```python
from build123d import *

# Parameters (mm, degrees)
F0_R     = 10
F2_DEPTH = 10
F1_R     = 6.465
F3_DEPTH = 12
F4_R     = 6.465
F6_DEPTH = 2
F7_D     = 10
F8_SIZE2 = 2
F8_SIZE  = 2
F9_SIZE2 = 0.5
F9_SIZE  = 0.5


with BuildPart() as f2:
    # F0 (on Top) → F2 (new body)
    with BuildSketch(Plane.XY):
        Circle(F0_R)
    extrude(amount=F2_DEPTH)

    # F1 (on Top) → F3 (cut)
    with BuildSketch(Plane.XY):
        Circle(F1_R)
    extrude(amount=F3_DEPTH, mode=Mode.SUBTRACT)

    # F4 (on face) → F6 (join)
    with BuildSketch(Plane.XY):
        Circle(F4_R)
    extrude(amount=F6_DEPTH)

    # F7 (through all)
    with Locations(Plane(origin=(0, 0, 0), x_dir=(1, 0, 0), z_dir=(0, 0, -1))):
        with Locations((0, 0)):
            Hole(F7_D / 2)

    # F8
    f8_edges = [f2.edges().sort_by_distance(p)[0] for p in [
        (-10, 0, 10),
        (-10, 0, 0),
    ]]
    chamfer(f8_edges, length=F8_SIZE, length2=F8_SIZE2)

    # F9
    f9_edges = [f2.edges().sort_by_distance(p)[0] for p in [
        (-6.465, 0, 10),
    ]]
    chamfer(f9_edges, length=F9_SIZE, length2=F9_SIZE2)


solid = f2.part
```
Here's how the part is built. I have some questions about the finished solid (model axes, mm). A direction names the side the tool comes from. Coordinates: 2 decimals unless noted, no trailing zeros. Order: outer loops, then holes, each group sorted by start corner. A loop starts at its lowest first (then second) coordinate and runs counter-clockwise, first axis right, second up. Notation, with made-up numbers: (-33.75, 18) - (1.25, 18) arc R29 ccw to (1.25, 42) - close; hole circle Ø6 at (41, -2.5). An arc over 180 degrees is marked (long way). One line per question, with ' | ' between items.
(1) Suppose I cut it at A-A on y = 0. List the corners of the cut face in (x, z) for me (3 decimals).
Report:
outline: (-10, 2) - (-8, 0) - (-5, 0) - (-5, 2) - (-6.465, 2) - (-6.465, 9.5) - (-6.965, 10) - (-8, 10) - (-10, 8) - close; (5, 0) - (8, 0) - (10, 2) - (10, 8) - (8, 10) - (6.965, 10) - (6.465, 9.5) - (6.465, 2) - (5, 2) - close
(2) If I drill on L1, parallel to Y at x = 0, z = 5.5 (3 decimals); L2, parallel to Y at x = 0, z = 1.05; L3, parallel to X at y = 5, z = 5.5, over which ranges is the centre line in solid material (lowest first)?
Report:
L1: y = -10 to -6.465, 6.465 to 10 | L2: y = -9.05 to -5, 5 to 9.05 | L3: x = -8.66 to -4.1, 4.1 to 8.66
(3) Will these pins go through, and if not, where does the flat tip stop? pin 1 (1 mm diameter, centred on y = -7.5, z = 6.5, fed in from +X); pin 2 (3 mm diameter, centred on x = -1, y = -4, fed in from +Z); pin 3 (2 mm diameter, centred on y = -4.5, z = 3, fed in from -X).
Report:
pin 1: stops at x = 7.14 | pin 2: stops at z = 2 | pin 3: stops at x = -9.37
(4) If we mould it in two halves opening along Y, with no side actions, what happens to faces 3 (the flat face through (2, -5, 2)), 4 (the conical face through (-1.06, 8.06, 0.13)), 5 (the flat face through (-2, 7, 10))? For each: pulls with the +Y half, pulls with the -Y half, needs draft (parallel to the pull), parting line crosses it, or undercut.
Report:
face 3: undercut | face 4: parting line crosses it | face 5: needs draft
(5) For faces 1 (the cylindrical face through (-1.4, -6.31, 5.7)), 2 (the cylindrical face through (1.08, 4.88, 1.01)), which set-ups out of +Z, -Z, +X, -X, +Y, -Y let a thin tool reach every point of the face, with its end or its side?
Report:
face 1: +Z | face 2: +Z, -Z
(6) Suppose I cut it at C-C on z = 4.5. List the corners of the cut face in (x, y) for me (3 decimals), and give its area (3 significant figures).
Report:
outline: circle Ø20 at (0, 0); hole circle Ø12.93 at (0, 0) | area: 183 mm2
